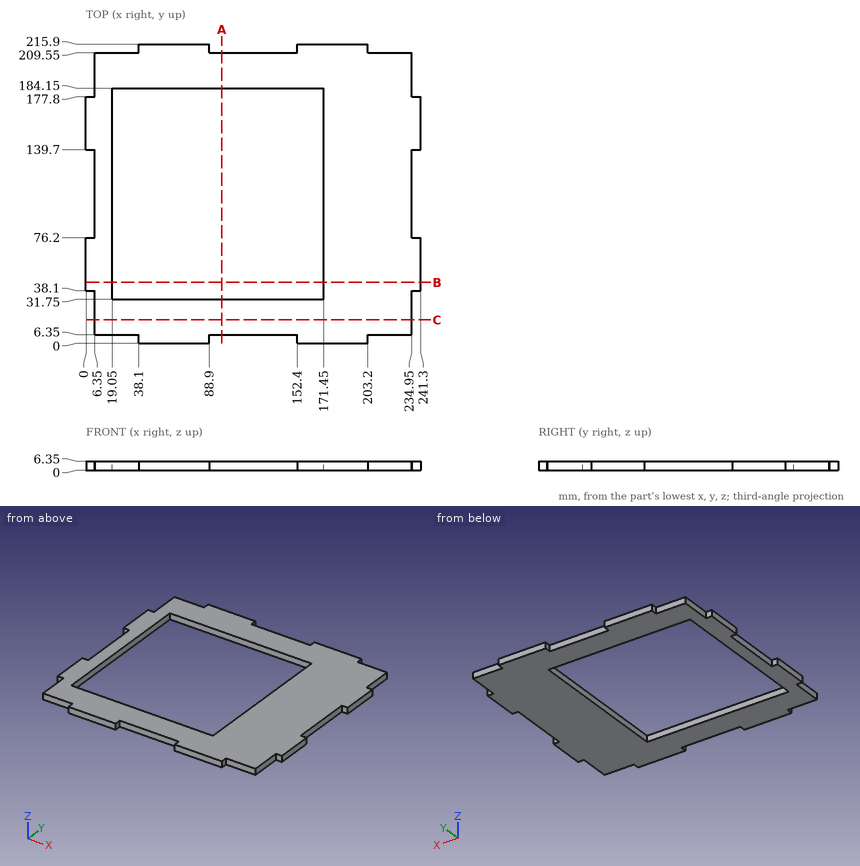
Input: dimensioned drawing with shaded views. Units: mm. Origin: part minimum x, y, z. Give positions to 0.01 mm unless a question says otherwise; leave off trailing zeros. Loops run counter-clockwise (first coordinate to the right, second up) from the corner with the lowest first, then second, coordinate; pieces in that order, holes last. Notation, with made-up numbers: M 65,8 L 104,8 A26 cw 104,33 Z; hole C -8,28 d6. An arc over 180 degrees is marked long. Put each result on its own line as item: value.
1) Cut plane B-B, the plane y = 44. Return the cut outline in (x, z), plus the area to 3 significant figures.
Computed values:
outline: M 0,0 L 19.05,0 L 19.05,6.35 L 0,6.35 Z; M 171.45,0 L 241.3,0 L 241.3,6.35 L 171.45,6.35 Z
area: 565 mm^2
2) Cut plane C-C, the plane y = 17. Return the cut outline in (x, z), plus the area to 3 significant figures.
Computed values:
outline: M 6.35,0 L 234.95,0 L 234.95,6.35 L 6.35,6.35 Z
area: 1,450 mm^2
3) Material intervals for L1, parallel to Y at x = 25, z = 5.75; L2, parallel to X at y = 135.5, z = 3; L3, parallel to X at y = 68, z = 4.25, sorted ascending. Write a range as from..to.
Computed values:
L1: y = 6.35..31.75, 184.15..209.55
L2: x = 6.35..19.05, 171.45..234.95
L3: x = 0..19.05, 171.45..241.3
4) First-contact query: P1, Ø3, axis at y = 22, z = 4.5, coming from the -X side; P2, Ø3, axis at y = 213.5, z = 2.5, coming from the +X side; P3, Ø1.5, axis at x = 134.5, z = 2.5, coming from the -Y side; P4, Ø3, axis at y = 44.5, z = 4, coming from the -X side. Flat tips, straight axial feed; report the tip coordinate or a pass-through.
Computed values:
P1: stops at x = 6.35
P2: stops at x = 203.2
P3: stops at y = 6.35
P4: stops at x = 0
5) Cut plane A-A, the plane x = 98. Return the cut outline in (y, z), plus the area to 3 significant figures.
Computed values:
outline: M 6.35,0 L 31.75,0 L 31.75,6.35 L 6.35,6.35 Z; M 184.15,0 L 209.55,0 L 209.55,6.35 L 184.15,6.35 Z
area: 323 mm^2
